Model file for the job. Use its own axes, mm. Face numbers are marked on the shaded views. A direction names the side the tool comes from. Round coordinates to 2 decimals unless told otherwise and drop trailing zeros. Loops run counter-clockwise (first coordinate to the right, second up) from the corner with the lowest first, then second, coordinate; pieces in that order, holes last. Notation, with made-up numbers: M 24,49 L 50,49 A23 cw 50,73 Z; hole C -12.75,-34 d1. An arc over 180 degrees is marked long. Use a Markdown table: item, result. Add a question column.
Q1. Probe line 1 (Z direction, x = -3, y = 10.5); line 2 (Y direction, x = 7, z = 1.85); line 3 (X direction, y = 8.5, z = 3.05). List the from-to ranges inside material, lowest first. Write a range as from..to.
Q2. Cut at D-D (z = 2.25). Give the cut face in (x, y).
Q3. Pin check, flat tip, straight feed: pin 1 (0.9 mm diameter, centred on x = 1.5, z = 2, fed in from +Y). Stop position of the tip, or through.
Q4. Cut at A-A (y = 10). Give the cut face in (x, z).
Q5. Mould opens along Z. For the marked faces 1, 2, 3 and 4 say: +Z half, -Z half, draft (parallel to the pull), parting line (faces both ways), or undercut.
Q6. Cut at C-C (y = 8.5). Give the cut face in (x, z).
Q7. Tool access for the marked faces 5 and 6: list every direction of +Z, -Z, +X, -X, +Y, -Y with a clear straight run to the whole face (end or side of a thin tool).
Q8. Cut at B-B (x = 4.75). Give the cut face in (y, z), plus the area to 3 significant figures.
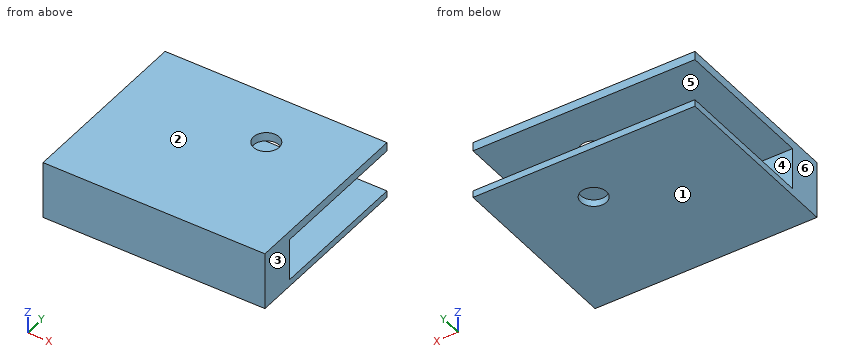
Autodesk Inventor part; units mm, degrees
ref_plane "YZ Plane" through (0, 0, 0) normal (1, 0, 0) x (0, 1, 0)
ref_plane "XZ Plane" through (0, 0, 0) normal (0, 1, 0) x (-1, 0, 0)
ref_plane "XY Plane" through (0, 0, 0) normal (0, 0, 1) x (1, 0, 0)
sketch "Sketch1" plane through (0, 0, 0) normal (0, 1, 0) x (-1, 0, 0)
  line L0 (0, 2.9392) -> (6.6347, 2.9392)
  line L1 (6.6347, 2.9392) -> (6.6347, 0)
  line L2 (6.6347, 0) -> (0, 0)
  line L3 (6.6347, 0) -> (6.6347, -0.4755)
  line L4 (6.6347, -0.4755) -> (0, -0.4755)
  line L5 (6.6347, 2.9392) -> (6.6347, 3.5443)
  line L6 (6.6347, 3.5443) -> (0, 3.5443)
  line L7 (0, 2.9392) -> (-8.8742, 2.9392)
  line L8 (-8.8742, 2.9392) -> (-8.8742, 0)
  line L9 (-8.8742, 0) -> (0, 0)
  line L10 (0, -0.4755) -> (-8.8742, -0.4755)
  line L11 (-8.8742, -0.4755) -> (-8.8742, 0)
  line L12 (0, 3.5443) -> (-8.8742, 3.5443)
  line L13 (-8.8742, 3.5443) -> (-8.8742, 2.9392)
extrude "Extrusion4" add sketch "Sketch1" along normal blind 12.7 contours L7 L13 L12 L6 L5 L0
extrude "Extrusion5" add sketch "Sketch1" along normal blind 12.7 contours L3 L4 L10 L11 L9 L2
extrude "Extrusion6" add sketch "Sketch1" along normal blind 2.54 contours L0 L1 L2 L9 L8 L7
sketch "Sketch2" plane through (8.8742, 0, -0.4755) normal (0, 0, -1) x (-1, 0, 0)
  circle A0 centre (5.8384, 8.836) radius 0.9005
  point P0 (8.8742, 0)
extrude "Extrusion7" cut sketch "Sketch2" against normal blind 25.4
properties part number "hook diagram"
Checked values:
| question | item | result |
|---|---|---|
| 1 | line 1 | z = -0.48..0, 2.94..3.54 |
| 1 | line 2 | y = 0..2.54 |
| 1 | line 3 | x = -6.63..2.2, 3.87..8.87 |
| 2 | outline | M -6.63,0 L 8.87,0 L 8.87,2.54 L -6.63,2.54 Z |
| 3 | pin 1 | stops at y = 2.54 |
| 4 | outline | M -6.63,-0.48 L 8.87,-0.48 L 8.87,0 L -6.63,0 Z; M -6.63,2.94 L 8.87,2.94 L 8.87,3.54 L -6.63,3.54 Z |
| 5 | face 1 | -Z half |
| 5 | face 2 | +Z half |
| 5 | face 3 | draft |
| 5 | face 4 | undercut |
| 6 | outline | M -6.63,-0.48 L 2.2,-0.48 L 2.2,0 L -6.63,0 Z; M -6.63,2.94 L 2.2,2.94 L 2.2,3.54 L -6.63,3.54 Z; M 3.87,-0.48 L 8.87,-0.48 L 8.87,0 L 3.87,0 Z; M 3.87,2.94 L 8.87,2.94 L 8.87,3.54 L 3.87,3.54 Z |
| 7 | face 5 | +X, -X, +Y |
| 7 | face 6 | +Z, -Z, -X, +Y, -Y |
| 8 | outline | M 0,-0.48 L 12.7,-0.48 L 12.7,0 L 2.54,0 L 2.54,2.94 L 12.7,2.94 L 12.7,3.54 L 0,3.54 Z |
| 8 | area | 21.2 mm^2 |
